Check sheet for the modelled part. Datum: model origin and axes. Units: mm. Face numbers are marked on the shaded views. A direction names the side the tool comes from. Round coordinates to 2 decimals unless told otherwise and drop trailing zeros. Order: outer loops, then holes, each group sorted by start corner. A loop starts at its lowest first (then second) coordinate and runs counter-clockwise, first axis right, second up.
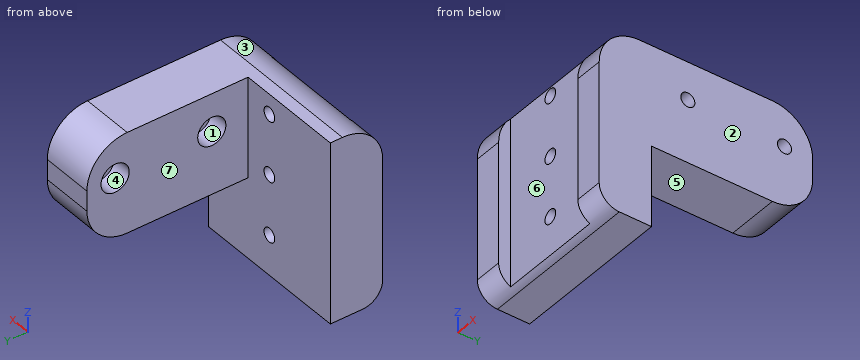
```python
from build123d import *

# Parameters (mm, degrees)
SKETCH1_W           = 40
SKETCH1_H           = 50
BOSS_EXTRUDE1_DEPTH = 13
SKETCH2_W           = 13
SKETCH2_H           = 30
BOSS_EXTRUDE2_DEPTH = 40
SKETCH3_R           = 1.75
CUT_EXTRUDE1_DEPTH  = 32
SKETCH4_W           = 26
SKETCH4_H           = 50
CUT_EXTRUDE2_DEPTH  = 3
SKETCH5_R           = 1.75
CUT_EXTRUDE3_DEPTH  = 10
SKETCH6_W           = 40
SKETCH6_H           = 53
CUT_EXTRUDE4_DEPTH  = 5
FILLET1_R           = 10
FILLET2_R           = 10
FILLET3_R           = 10
FILLET4_R           = 5
SKETCH7_R           = 3.5
CUT_EXTRUDE5_DEPTH  = 5


with BuildPart() as part:
    # Sketch1 → Boss-Extrude1 (new body)
    with BuildSketch(Plane(origin=(0, 0, 0), x_dir=(1, 0, 0), z_dir=(0, 1, 0))):
        Rectangle(SKETCH1_W, SKETCH1_H)
    extrude(amount=BOSS_EXTRUDE1_DEPTH)

    # Sketch2 → Boss-Extrude2 (add)
    with BuildSketch(Plane(origin=(0, 13, 0), x_dir=(1, 0, 0), z_dir=(0, 1, 0))):
        with Locations((13.5, -10)):
            Rectangle(SKETCH2_W, SKETCH2_H)
    extrude(amount=BOSS_EXTRUDE2_DEPTH)

    # Sketch3 → Cut-Extrude1 (cut)
    with BuildSketch(Plane(origin=(20, 0, 0), x_dir=(0, 0, -1), z_dir=(1, 0, 0))):
        with Locations((-10, 46)):
            Circle(SKETCH3_R)
        with Locations((-10.616810137, 22)):
            Circle(SKETCH3_R)
    extrude(amount=-CUT_EXTRUDE1_DEPTH, mode=Mode.SUBTRACT)

    # Sketch4 → Cut-Extrude2 (cut)
    with BuildSketch(Plane(origin=(0, 0, 0), x_dir=(-1, 0, 0), z_dir=(0, -1, 0))):
        Rectangle(SKETCH4_W, SKETCH4_H)
    extrude(amount=-CUT_EXTRUDE2_DEPTH, mode=Mode.SUBTRACT)

    # Sketch5 → Cut-Extrude3 (cut)
    with BuildSketch(Plane(origin=(0, 3, 0), x_dir=(-1, 0, 0), z_dir=(0, -1, 0))):
        with Locations(Location((0, 0, 0), (0, 0, 90))):
            Circle(SKETCH5_R)
        with Locations(Location((0, -15, 0), (0, 0, 90))):
            Circle(SKETCH5_R)
        with Locations(Location((0, 15, 0), (0, 0, 90))):
            Circle(SKETCH5_R)
    extrude(amount=-CUT_EXTRUDE3_DEPTH, mode=Mode.SUBTRACT)

    # Sketch6 → Cut-Extrude4 (cut)
    with BuildSketch(Plane.XY.offset(25)):
        with Locations((0, 26.5)):
            Rectangle(SKETCH6_W, SKETCH6_H)
    extrude(amount=-CUT_EXTRUDE4_DEPTH, mode=Mode.SUBTRACT)

    # Fillet1
    fillet1_edges = [part.edges().sort_by_distance(p)[0] for p in [
        (13.5, 53, 20),
    ]]
    fillet(fillet1_edges, radius=FILLET1_R)

    # Fillet2
    fillet2_edges = [part.edges().sort_by_distance(p)[0] for p in [
        (13.5, 53, -5),
    ]]
    fillet(fillet2_edges, radius=FILLET2_R)

    # Fillet3
    fillet3_edges = [part.edges().sort_by_distance(p)[0] for p in [
        (-16.5, 0, 20),
    ]]
    fillet(fillet3_edges, radius=FILLET3_R)

    # Fillet4
    fillet4_edges = [part.edges().sort_by_distance(p)[0] for p in [
        (-16.5, 0, -25),
    ]]
    fillet(fillet4_edges, radius=FILLET4_R - 0.0001)  # a hair under: the kernel refuses the full size

    # Sketch7 → Cut-Extrude5 (cut)
    with BuildSketch(Plane.ZY.offset(-7)):
        with Locations((10.616810137, 22)):
            Circle(SKETCH7_R)
        with Locations((10, 46)):
            Circle(SKETCH7_R)
    extrude(amount=-CUT_EXTRUDE5_DEPTH, mode=Mode.SUBTRACT)


solid = part.part
```
Item 1: Go/stop test with flat-tipped pins: P1, Ø12.5, axis at y = 31, z = 5, coming from the -X side; P2, Ø3, axis at x = 0, z = 15, coming from the +Y side; P3, Ø4, axis at x = 9, y = 45, coming from the -Z side; P4, Ø13, axis at x = -4.5, z = 3, coming from the -Y side. Record where each tip stops, or that it passes through.
Answer:
P1: stops at x = 7
P2: passes through
P3: stops at z = -5
P4: stops at y = 3
Item 2: Sectioned sample at D-D (x = 0). Record the cut outline in (y, z).
Answer:
outline: (3, -24.58) arc R5 ccw to (5, -25) - (13, -25) - (13, -16.75) - (3, -16.75) - close; (3, -13.25) - (13, -13.25) - (13, -1.75) - (3, -1.75) - close; (3, 1.75) - (13, 1.75) - (13, 13.25) - (3, 13.25) - close; (3, 16.75) - (13, 16.75) - (13, 20) - (10, 20) arc R10 ccw to (3, 17.14) - close
Item 3: Sectioned sample at B-B (y = 22). Record the cut outline in (x, z).
Answer:
outline: (7, -5) - (20, -5) - (20, 8.87) - (12, 8.87) - (12, 7.12) - (7, 7.12) - close; (7, 14.12) - (12, 14.12) - (12, 12.37) - (20, 12.37) - (20, 20) - (7, 20) - close
Item 4: Scan lines: line 1 along X through (y, z) = (6.25, 15); line 2 along Y through (x, z) = (0, -22.5); line 3 along X through (y, z) = (24, 15.5). Record each from-to range of solid material in increasing order.
Answer:
line 1: x = -20 to -1.75, 1.75 to 20
line 2: y = 3 to 13
line 3: x = 7 to 20
Item 5: Sectioned sample at A-A (z = -15). Record the cut outline in (x, y).
Answer:
outline: (-20, 0) - (-13, 0) - (-13, 3) - (-1.75, 3) - (-1.75, 13) - (-20, 13) - close; (1.75, 3) - (13, 3) - (13, 0) - (20, 0) - (20, 13) - (1.75, 13) - close
Item 6: Access from +Z, -Z, +X, -X, +Y, -Y to the whole of each face (thin tool, end or side, straight path). Record for the marked faces 4, 5, 6 and 7.
Answer:
face 4: -X
face 5: -Z, +X, -X, +Y
face 6: +Z, -Z, -Y
face 7: +Z, -Z, -X, +Y
Item 7: Release check for a two-part mould opening along Y. For the marked faces 1, 2 and 3 record: released by +Y, released by -Y, zero draft, split by the parting line, or undercut.
Answer:
face 1: undercut
face 2: zero draft
face 3: released by -Y
Item 8: Sectioned sample at C-C (x = 15). Record the cut outline in (y, z), and give its area (3 significant figures).
Answer:
outline: (0, -20) arc R5 ccw to (5, -25) - (13, -25) - (13, -5) - (43, -5) arc R10 ccw to (53, 5) - (53, 10) arc R10 ccw to (43, 20) - (10, 20) arc R10 ccw to (0, 10) - close; hole circle Ø3.5 at (22, 10.62); hole circle Ø3.5 at (46, 10)
area: 1,500 mm2
